Here's how the part is built. I have some questions about the finished solid (model axes, mm). A direction names the side the tool comes from. Round coordinates to 2 decimals unless told otherwise and drop trailing zeros. Write each loop counter-clockwise with the first axis right and the second up, starting at its lowest first coordinate (ties: lowest second). Pieces come first, ordered by that corner, then holes. Notation, with made-up numbers: (-5, 53) -> (1, 53) arc R10 cw to (1, 64) -> close; hole circle Ø5 at (-27.5, -40). An arc over 180 degrees is marked (long way). Answer as CSV lines item,"result".
```python
from build123d import *

# Parameters (mm, degrees)
SKETCH1_R           = 5
BOSS_EXTRUDE1_DEPTH = 15
SKETCH7_W           = 1.25
SKETCH7_H           = 2.348715111


with BuildPart() as part:
    # Sketch1 → Boss-Extrude1 (new body)
    with BuildSketch(Plane.XY):
        with BuildLine():
            ThreePointArc((10.519556214, -1.031424774), (10.557381521, -0.516328781), (10.57, 0))
            ThreePointArc((10.57, 0), (10.557381521, 0.516328781), (10.519556214, 1.031424774))
            ThreePointArc((10.519556214, 1.031424774), (8.257639416, 1.884752311), (9.92531109, 3.634982773))
            ThreePointArc((9.92531109, 3.634982773), (9.523240934, 4.586151122), (9.030274215, 5.493545995))
            ThreePointArc((9.030274215, 5.493545995), (6.622112657, 5.280958622), (7.36523638, 7.581437401))
            ThreePointArc((7.36523638, 7.581437401), (6.590287206, 8.26395877), (5.752435659, 8.867603058))
            ThreePointArc((5.752435659, 8.867603058), (3.67499527, 7.631206311), (3.346386275, 10.026295373))
            ThreePointArc((3.346386275, 10.026295373), (2.352046272, 10.304988032), (1.335256672, 10.485322581))
            ThreePointArc((1.335256672, 10.485322581), (1.421024661, 10.208424883), (1.45, 9.92))
            ThreePointArc((1.45, 9.92), (-0.288424883, 8.498975339), (-1.335256672, 10.485322581))
            ThreePointArc((-1.335256672, 10.485322581), (-2.352046272, 10.304988032), (-3.346386275, 10.026295373))
            ThreePointArc((-3.346386275, 10.026295373), (-2.98291066, 9.535012373), (-2.854126692, 8.93761117))
            ThreePointArc((-2.854126692, 8.93761117), (-4.269112426, 7.488033989), (-5.752435659, 8.867603058))
            ThreePointArc((-5.752435659, 8.867603058), (-6.590287206, 8.26395877), (-7.36523638, 7.581437401))
            ThreePointArc((-7.36523638, 7.581437401), (-6.600612193, 7.061440168), (-6.305768306, 6.185018834))
            ThreePointArc((-6.305768306, 6.185018834), (-7.399070653, 4.779576988), (-9.030274215, 5.493545995))
            ThreePointArc((-9.030274215, 5.493545995), (-9.523240934, 4.586151122), (-9.92531109, 3.634982773))
            ThreePointArc((-9.92531109, 3.634982773), (-8.740113044, 3.318901703), (-8.221284889, 2.207407665))
            ThreePointArc((-8.221284889, 2.207407665), (-9.010790158, 0.916575875), (-10.519556214, 1.031424774))
            ThreePointArc((-10.519556214, 1.031424774), (-10.57, 0), (-10.519556214, -1.031424774))
            ThreePointArc((-10.519556214, -1.031424774), (-9.010790158, -0.916575875), (-8.221284889, -2.207407665))
            ThreePointArc((-8.221284889, -2.207407665), (-8.740113044, -3.318901703), (-9.92531109, -3.634982773))
            ThreePointArc((-9.92531109, -3.634982773), (-9.523240934, -4.586151122), (-9.030274215, -5.493545995))
            ThreePointArc((-9.030274215, -5.493545995), (-7.399070653, -4.779576988), (-6.305768306, -6.185018834))
            ThreePointArc((-6.305768306, -6.185018834), (-6.600612193, -7.061440168), (-7.36523638, -7.581437401))
            ThreePointArc((-7.36523638, -7.581437401), (-6.590287206, -8.26395877), (-5.752435659, -8.867603058))
            ThreePointArc((-5.752435659, -8.867603058), (-4.269112426, -7.488033989), (-2.854126692, -8.93761117))
            ThreePointArc((-2.854126692, -8.93761117), (-2.98291066, -9.535012373), (-3.346386275, -10.026295373))
            ThreePointArc((-3.346386275, -10.026295373), (-2.352046272, -10.304988032), (-1.335256672, -10.485322581))
            ThreePointArc((-1.335256672, -10.485322581), (-0.288424883, -8.498975339), (1.45, -9.92))
            ThreePointArc((1.45, -9.92), (1.421024661, -10.208424883), (1.335256672, -10.485322581))
            ThreePointArc((1.335256672, -10.485322581), (2.352046272, -10.304988032), (3.346386275, -10.026295373))
            ThreePointArc((3.346386275, -10.026295373), (3.67499527, -7.631206311), (5.752435659, -8.867603058))
            ThreePointArc((5.752435659, -8.867603058), (6.590287206, -8.26395877), (7.36523638, -7.581437401))
            ThreePointArc((7.36523638, -7.581437401), (6.622112657, -5.280958622), (9.030274215, -5.493545995))
            ThreePointArc((9.030274215, -5.493545995), (9.523240934, -4.586151122), (9.92531109, -3.634982773))
            ThreePointArc((9.92531109, -3.634982773), (8.257639416, -1.884752311), (10.519556214, -1.031424774))
        make_face()
        Circle(SKETCH1_R, mode=Mode.SUBTRACT)
    extrude(amount=BOSS_EXTRUDE1_DEPTH)

    # Sketch7 → M3 Tapped Hole1 (revolve, cut)
    with BuildSketch(Plane(origin=(8.221284889, -2.134982773, 6.95), x_dir=(0, 0, 1), z_dir=(0, 1, 0))):
        with Locations((0.625, 1.174357556)):
            Rectangle(SKETCH7_W, SKETCH7_H)
    revolve(axis=Axis((1.871284889, -2.134982773, 6.95), (1, 0, 0)), mode=Mode.SUBTRACT)


solid = part.part
```
1. Suppose I cut it at C-C on y = 1.5. Please give me the cut outline in (x, z).
Numbers:
outline,"(-8.41, 0) -> (-4.77, 0) -> (-4.77, 15) -> (-8.41, 15) -> close; (4.77, 0) -> (8.41, 0) -> (8.41, 15) -> (4.77, 15) -> close"
2. Suppose I cut it at B-B on x = 7. Please give me the cut outline in (y, z).
Numbers:
outline,"(-7.92, 0) -> (-7.42, 0) -> (-7.42, 15) -> (-7.92, 15) -> close; (-4.95, 0) -> (4.95, 0) -> (4.95, 15) -> (-4.95, 15) -> close; (7.42, 0) -> (7.92, 0) -> (7.92, 15) -> (7.42, 15) -> close"
3. If we mould it in two halves opening along Y, with no side actions, what happens to faces 1 (the face through (-9.517, 4.599, 7.395)), 2 (the face through (8.267, 1.846, 7.395)), 3 (the face through (6.58, -8.27, 7.4))? For each: released by +Y, released by -Y, zero draft, split by the parting line, or undercut.
Numbers:
face 1,"released by +Y"
face 2,"undercut"
face 3,"released by -Y"
4. On a 3-axis mill with a long thin cutter (end or side, diameter ignored), from which of +Z, -Z, +X, -X, +Y, -Y can I reach the whole of each face in a straight line? I mean faces 4 (the face through (8.46, -3.385, 6.977)), 5 (the face through (2.37, 10.3, 7.4)). Say none if no direction works.
Numbers:
face 4,"+X"
face 5,"+Z, -Z, +X, +Y"
5. If I drill on line 1 (Y direction, x = -9.5, z = 7.5); line 2 (Y direction, x = -8.75, z = 11.25); line 3 (Y direction, x = 0, z = 9.5), over which ranges is the centre line in solid material (lowest first)?
Numbers:
line 1,"y = -4.63 to -3.65, -0.77 to 0.77, 3.65 to 4.63"
line 2,"y = -5.13 to -3.33, -1.09 to 1.09, 3.33 to 5.13"
line 3,"y = -8.47 to -5, 5 to 8.47"
6. Suppose I cut it at A-A on x = 0. Please give me the cut outline in (y, z).
Numbers:
outline,"(-8.47, 0) -> (-5, 0) -> (-5, 15) -> (-8.47, 15) -> close; (5, 0) -> (8.47, 0) -> (8.47, 15) -> (5, 15) -> close"
7. For pin 1 Ø4 at (x, y) = (0, 9.92) entering from -Z; pin 2 Ø2 at (y, z) = (-6, 3.5) entering from -X; pin 3 Ø8 at (x, z) = (-7.5, 3.5) entering from -Y; pin 4 Ø5 at (x, z) = (2.5, 8) entering from +Y, each with a flat end and sliding along its axis, tell me the tip position at first contact or that it passes through.
Numbers:
pin 1,"stops at z = 0"
pin 2,"stops at x = -9.31"
pin 3,"stops at y = -8.87"
pin 4,"stops at y = 10.49"
8. Suppose I cut it at D-D on y = -6.75. Please give me the cut outline in (x, z), and give its area (3 significant figures).
Numbers:
outline,"(-6.42, 0) -> (6.42, 0) -> (6.42, 15) -> (-6.42, 15) -> close"
area,"193 mm^2"
